```python
from build123d import *

# Parameters (mm, degrees)
BOSS_EXTRUDE1_DEPTH = 10.16
SKETCH2_R           = 12.7
CUT_EXTRUDE1_DEPTH  = 5.08
BOSS_EXTRUDE2_DEPTH = 10.16


with BuildPart() as part:
    # Sketch1 → Boss-Extrude1 (new body)
    with BuildSketch(Plane(origin=(0, 0, 0), x_dir=(1, 0, 0), z_dir=(0, 1, 0))):
        Polygon((38.1, 65.991135768), (-38.1, 65.991135768), (-76.2, 0), (-38.1, -65.991135768), (38.1, -65.991135768), (76.2, 0), align=None)
    boss_extrude1 = extrude(amount=BOSS_EXTRUDE1_DEPTH)

    # Sketch2 → Cut-Extrude1 (cut)
    with BuildSketch(Plane(origin=(0, 10.16, 0), x_dir=(1, 0, 0), z_dir=(0, 1, 0))):
        with Locations((-50.8, 0)):
            Circle(SKETCH2_R)
        with Locations((50.8, 0)):
            Circle(SKETCH2_R)
    cut_extrude1 = extrude(amount=-CUT_EXTRUDE1_DEPTH, mode=Mode.SUBTRACT)

    # Mirror1: Boss-Extrude1, Cut-Extrude1 across plane
    add(boss_extrude1.mirror(Plane(origin=(76.2, 10.16, 0), x_dir=(0.5, 0, 0.866025404), z_dir=(-0.866025404, 0, 0.5))))
    add(cut_extrude1.mirror(Plane(origin=(76.2, 10.16, 0), x_dir=(0.5, 0, 0.866025404), z_dir=(-0.866025404, 0, 0.5))), mode=Mode.SUBTRACT)

    # Sketch3 → Boss-Extrude2 (add)
    with BuildSketch(Plane(origin=(0, 10.16, 0), x_dir=(1, 0, 0), z_dir=(0, 1, 0))):
        Polygon((12.7, 21.997045256), (-12.7, 21.997045256), (-25.4, 0), (-12.7, -21.997045256), (12.7, -21.997045256), (25.4, 0), align=None)
    boss_extrude2 = extrude(amount=BOSS_EXTRUDE2_DEPTH)

    # Mirror2: Boss-Extrude2 across plane
    add(boss_extrude2.mirror(Plane(origin=(57.15, 0, -32.995567884), x_dir=(0.5, 0, 0.866025404), z_dir=(0.866025404, 0, -0.5))))


solid = part.part
```
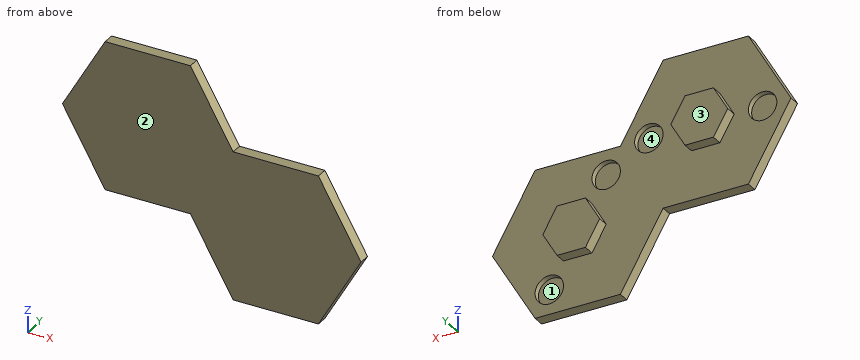
Build history of the part. All positions in model axes, mm. Face numbers are marked on the shaded views. A direction names the side the tool comes from. Round coordinates to 2 decimals unless told otherwise and drop trailing zeros. Order: outer loops, then holes, each group sorted by start corner. A loop starts at its lowest first (then second) coordinate and runs counter-clockwise, first axis right, second up. Notation, with made-up numbers: (-13, 88) -> (0, 88) arc R24 ccw to (0, 126) -> close; hole circle Ø5 at (-16.5, 43). An arc over 180 degrees is marked (long way). Answer in a Markdown table with one row per item.
1) Pin check, flat tips, straight feed: P1, Ø3, axis at x = 4, y = 16, coming from the -Z side; P2, Ø6, axis at x = 153.5, z = -8.5, coming from the +Y side; P3, Ø20.5, axis at x = 139.7, z = -109.99, coming from the -Y side; P4, Ø5, axis at x = -2.5, y = 14.5, coming from the +Z side. Stop position of each tip, or through.
Values:
| item | result |
|---|---|
| P1 | z = -22 |
| P2 | y = 10.16 |
| P3 | y = 0 |
| P4 | z = 22 |
2) Band-saw the part on A-A on y = 15. Give the cut face in (x, z).
Values:
| item | result |
|---|---|
| outline | (-25.4, 0) -> (-12.7, -22) -> (12.7, -22) -> (25.4, 0) -> (12.7, 22) -> (-12.7, 22) -> close; (88.9, -65.99) -> (101.6, -87.99) -> (127, -87.99) -> (139.7, -65.99) -> (127, -43.99) -> (101.6, -43.99) -> close |
3) Which spindle directions (+Z, -Z, +X, -X, +Y, -Y) get a long thin tool onto all of the face, cutting with end or side? Do the marked faces 1 and 2. Say none if no direction does.
Values:
| item | result |
|---|---|
| face 1 | +Y |
| face 2 | +Z, -Z, +X, -X, -Y |
4) Mould opens along X. For the marked faces 3 and 4 say: released by +X, released by -X, zero draft, split by the parting line, or undercut.
Values:
| item | result |
|---|---|
| face 3 | zero draft |
| face 4 | undercut |
5) Band-saw the part on C-C on z = 18. Give the cut face in (x, y).
Values:
| item | result |
|---|---|
| outline | (-65.81, 0) -> (65.81, 0) -> (65.81, 10.16) -> (15.01, 10.16) -> (15.01, 20.32) -> (-15.01, 20.32) -> (-15.01, 10.16) -> (-65.81, 10.16) -> close |
6) Band-saw the part on B-B on x = 124. Give the cut face in (y, z).
Values:
| item | result |
|---|---|
| outline | (0, -131.98) -> (10.16, -131.98) -> (10.16, -87.99) -> (20.32, -87.99) -> (20.32, -43.99) -> (10.16, -43.99) -> (10.16, 0) -> (0, 0) -> close |
7) Wall check: L1, parallel to Z at x = 139.7, y = 7.55; L2, parallel to X at y = 9.25, z = 11.5; L3, parallel to Y at x = 141.5, z = -42. Give the ranges that are in metal, low to high.
Values:
| item | result |
|---|---|
| L1 | -131.98 to -122.69, -97.29 to 0 |
| L2 | -69.56 to -56.19, -45.41 to 45.41, 56.19 to 69.56 |
| L3 | 0 to 10.16 |
8) Band-saw the part on D-D on z = -41. Give the cut face in (x, y).
Values:
| item | result |
|---|---|
| outline | (-52.53, 0) -> (176.07, 0) -> (176.07, 10.16) -> (-52.53, 10.16) -> close |
